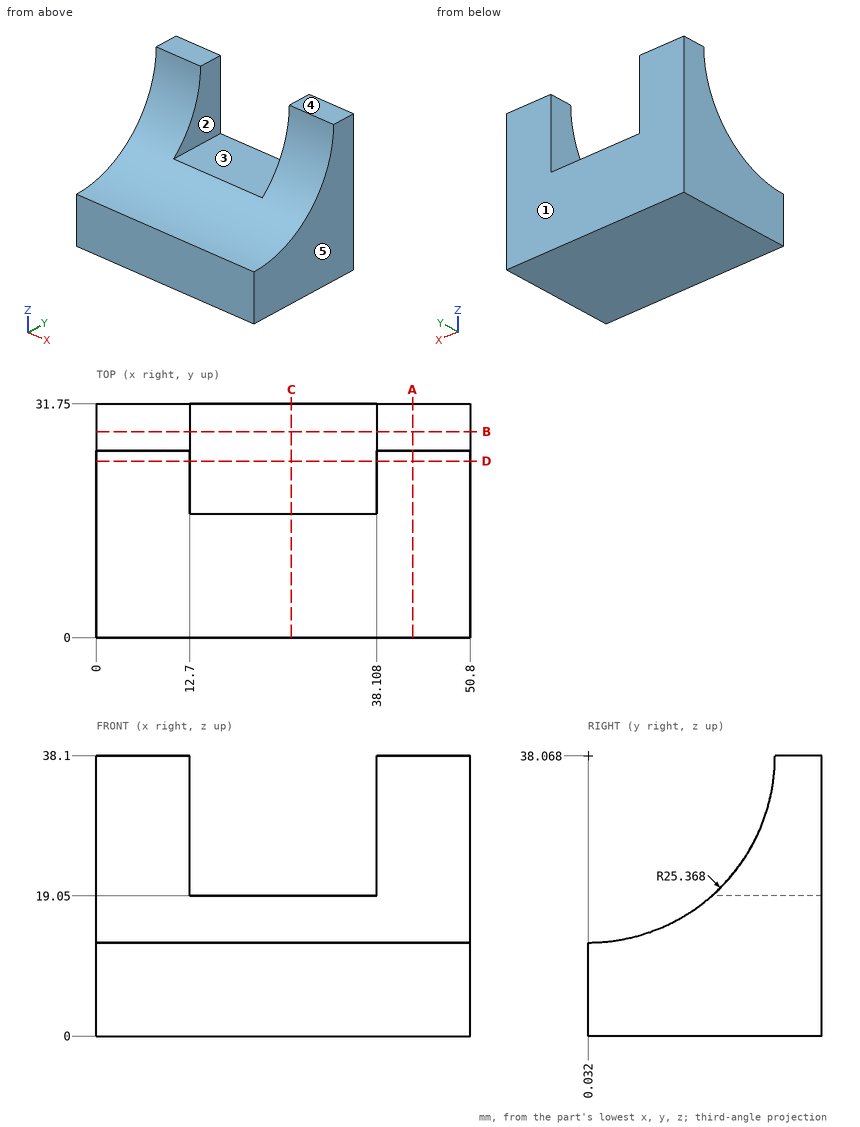
Drawing for the job (mm, zero at the part's lowest x, y, z). A direction names the side the tool comes from. Round coordinates to 2 decimals unless told otherwise and drop trailing zeros. Order: outer loops, then holes, each group sorted by start corner. A loop starts at its lowest first (then second) coordinate and runs counter-clockwise, first axis right, second up. Notation, with made-up numbers: M -16.5,20.25 L -10.5,20.25 A13 ccw -10.5,28.25 Z; hole C 44.5,1.5 d1. An arc over 180 degrees is marked long. Use one line per item in the form item = value.
Q1. Saw through at B-B on y = 28. Give the cut face in (x, z), then the cut area to 3 significant figures.
Recorded:
outline = M 0,0 L 50.8,0 L 50.8,38.1 L 38.11,38.1 L 38.11,19.05 L 12.7,19.05 L 12.7,38.1 L 0,38.1 Z
area = 1,450 mm^2
Q2. Probe L1, parallel to X at y = 23, z = 27; L2, parallel to Z at x = 21.5, y = 20; L3, parallel to Y at x = 48.5, z = 20. List the from-to ranges inside material, lowest first.
Recorded:
L1 = 0 to 12.7, 38.11 to 50.8
L2 = 0 to 19.05
L3 = 17.84 to 31.75
Q3. Saw through at A-A on x = 43. Give the cut face in (y, z).
Recorded:
outline = M 0,0 L 31.75,0 L 31.75,38.1 L 25.4,38.1 A25.37 cw 0,12.7 Z
Q4. Saw through at C-C on x = 26.5. Give the cut face in (y, z).
Recorded:
outline = M 0,0 L 31.75,0 L 31.75,19.05 L 16.82,19.05 A25.37 cw 0,12.7 Z
Q5. Two-plate mould, pull along X, no slides. Class the marked faces 3, 4 and 5: +X half, -X half, draft (parallel to the pull), parting line (faces both ways), or undercut.
Recorded:
face_3 = undercut
face_4 = draft
face_5 = +X half
Q6. Flat gauge pins, fed straight in: P1, Ø3, axis at y = 26.5, z = 5, coming from the -X side; P2, Ø5, axis at y = 10.5, z = 19, coming from the +X side; P3, Ø4.5, axis at x = 26, y = 27.5, coming from the +Z side; P4, Ø3, axis at x = 39.5, z = 24.5, coming from the -Y side. Where does each tip first touch, or does it go through?
Recorded:
P1 = 0
P2 = through
P3 = 19.05
P4 = 20.44
Q7. Which spindle directions (+Z, -Z, +X, -X, +Y, -Y) get a long thin tool onto all of the face, cutting with end or side? Do the marked faces 1 and 2. Say none if no direction does.
Recorded:
face_1 = +Z, -Z, +X, -X, +Y
face_2 = +Z, +Y, -Y
Q8. Saw through at D-D on y = 24. Give the cut face in (x, z).
Recorded:
outline = M 0,0 L 50.8,0 L 50.8,29.76 L 38.11,29.76 L 38.11,19.05 L 12.7,19.05 L 12.7,29.76 L 0,29.76 Z
